Source: CAD feature listing. Evaluate the final solid. Frame: model axes, mm. Face numbers are marked on the shaded views. A direction names the side the tool comes from. Give positions to 0.01 mm unless a question says otherwise; leave off trailing zeros. Write each loop counter-clockwise with the first axis right and the second up, starting at its lowest first coordinate (ties: lowest second). Pieces come first, ordered by that corner, then holes. Notation, with made-up numbers: (57, -8) -> (88, -8) arc R22 ccw to (88, 11) -> close; hole circle Ø11 at (46, 74). An arc over 180 degrees is marked (long way). Use one line per item in the form item = value. Start each with the question number.
(1) Draft query along Z for the marked faces 4 and 5. Return one class per face: pulls with the +Z half, pulls with the -Z half, needs draft (parallel to the pull), parting line crosses it, or undercut.
(2) Cut plane A-A, the plane y = -1.25. Output: boundary loops of the cut face in (x, z), and give its area (3 significant figures).
(3) Material intervals for line 1 along Z through (x, y) = (-51, 4.75); line 2 along X through (y, z) = (7.25, -16); line 3 along X through (y, z) = (8.25, -3), sorted ascending. Write a range as from..to.
(4) Cut plane B-B, the plane x = 36.5. Output: boundary loops of the cut face in (y, z), and give its area (3 significant figures).
(5) First-contact query: P1, Ø2.5, axis at x = -8.5, y = -1.5, coming from the +Z side; P2, Ø2.5, axis at y = 1.5, z = 25, coming from the -X side; P3, Ø0.9, axis at x = -5.5, y = -2, coming from the -Z side. Flat tips, straight axial feed; report the tip coordinate or a pass-through.
(6) Cut plane C-C, the plane z = 11. Output: boundary loops of the cut face in (x, y).
(7) Cut plane D-D, the plane y = 6. Output: boundary loops of the cut face in (x, z).
(8) Set-up query: the marked faces 1, 2 and 3. Return all of +Z, -Z, +X, -X, +Y, -Y with unobstructed straight access to the full face (end or side cutting, diameter ignored); none if empty.
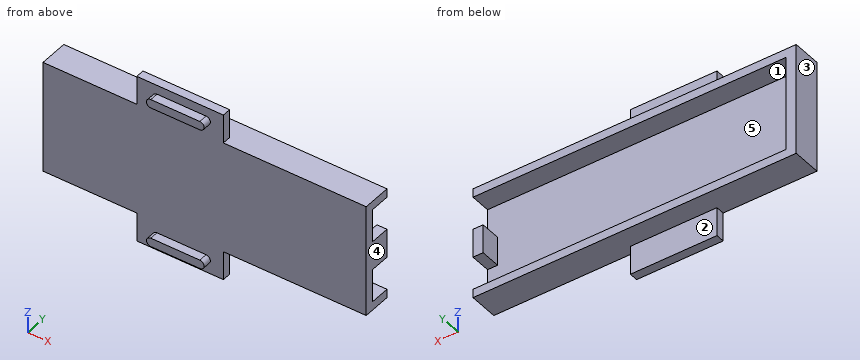
from build123d import *

# Parameters (mm, degrees)
SKETCH1_W           = 112
SKETCH1_H           = 39
SKETCH1_W_2         = 105
SKETCH1_H_2         = 33
BOSS_EXTRUDE1_DEPTH = 10
SKETCH2_W           = 105
SKETCH2_H           = 33
BOSS_EXTRUDE2_DEPTH = 3
SKETCH3_W           = 11.5
SKETCH3_H           = 10.919197496
SKETCH3_H_2         = 11.051284563
CUT_EXTRUDE1_DEPTH  = 111.691011379
SKETCH4_W           = 30
SKETCH4_H           = 10
BOSS_EXTRUDE3_DEPTH = 3
SKETCH5_W           = 17
SKETCH5_H           = 3
BOSS_EXTRUDE4_DEPTH = 3


with BuildPart() as part:
    # Sketch1 → Boss-Extrude1 (new body)
    with BuildSketch(Plane(origin=(0, 0, 0), x_dir=(1, 0, 0), z_dir=(0, 1, 0))):
        Rectangle(SKETCH1_W, SKETCH1_H)
        Rectangle(SKETCH1_W_2, SKETCH1_H_2, mode=Mode.SUBTRACT)
    extrude(amount=BOSS_EXTRUDE1_DEPTH)

    # Sketch2 → Boss-Extrude2 (add)
    with BuildSketch(Plane(origin=(0, 0, 0), x_dir=(1, 0, 0), z_dir=(0, 1, 0))):
        Rectangle(SKETCH2_W, SKETCH2_H)
    extrude(amount=BOSS_EXTRUDE2_DEPTH)

    # Sketch3 → Cut-Extrude1 (cut, through all)
    with BuildSketch(Plane.ZY.offset(-52.5)):
        with Locations((-10.75, 8.459598748)):
            Rectangle(SKETCH3_W, SKETCH3_H)
        with Locations((10.75, 8.525642282)):
            Rectangle(SKETCH3_W, SKETCH3_H_2)
    extrude(amount=-CUT_EXTRUDE1_DEPTH, mode=Mode.SUBTRACT)

    # Sketch4 → Boss-Extrude3 (add)
    with BuildSketch(Plane(origin=(0, 0, 0), x_dir=(1, 0, 0), z_dir=(0, 1, 0))):
        with Locations((-8.5, 24.5)):
            Rectangle(SKETCH4_W, SKETCH4_H)
        with Locations((-8.5, -24.5)):
            Rectangle(SKETCH4_W, SKETCH4_H)
    extrude(amount=BOSS_EXTRUDE3_DEPTH)

    # Sketch5 → Boss-Extrude4 (add)
    with BuildSketch(Plane.XZ):
        with Locations((-8, 24.845915891)):
            Rectangle(SKETCH5_W, SKETCH5_H)
        with BuildLine():
            Line((-16.5, 26.345915891), (-16.5, 23.345915891))
            ThreePointArc((-16.5, 23.345915891), (-18, 24.845915891), (-16.5, 26.345915891))
        make_face()
        with BuildLine():
            ThreePointArc((0.5, 26.345915891), (2, 24.845915891), (0.5, 23.345915891))
            Line((0.5, 23.345915891), (0.5, 26.345915891))
        make_face()
    boss_extrude4 = extrude(amount=BOSS_EXTRUDE4_DEPTH)

    # Mirror1: Boss-Extrude4 across plane
    add(boss_extrude4.mirror(Plane.XY))


solid = part.part
Geometry says:
q1.face_4 = needs draft
q1.face_5 = undercut
q2.outline = (-16.5, -26.35) -> (0.5, -26.35) arc R1.5 ccw to (0.5, -23.35) -> (-16.5, -23.35) arc R1.5 ccw to start; (-16.5, 23.35) -> (0.5, 23.35) arc R1.5 ccw to (0.5, 26.35) -> (-16.5, 26.35) arc R1.5 ccw to start
q2.area = 116 mm^2
q3.line_1 = -19.5..-16.5, 16.5..19.5
q3.line_2 = -56..-52.5
q3.line_3 = -56..-52.5, 52.5..56
q4.outline = (0, -19.5) -> (10, -19.5) -> (10, -16.5) -> (3, -16.5) -> (3, 16.5) -> (10, 16.5) -> (10, 19.5) -> (0, 19.5) -> close
q4.area = 159 mm^2
q5.P1 = 26.35
q5.P2 = -23.5
q5.P3 = -26.35
q6.outline = (-56, 0) -> (56, 0) -> (56, 3) -> (-52.5, 3) -> (-52.5, 10) -> (-56, 10) -> close
q7.outline = (-56, -19.5) -> (56, -19.5) -> (56, -16.5) -> (-52.5, -16.5) -> (-52.5, 16.5) -> (56, 16.5) -> (56, 19.5) -> (-56, 19.5) -> close; (52.5, -5) -> (56, -5) -> (56, 5) -> (52.5, 5) -> close
q8.face_1 = +X, +Y
q8.face_2 = -Z, +X, -X, +Y
q8.face_3 = +Z, -Z, -X, +Y, -Y
